Geometry check sheet. Reference: drawing and pictorial views, mm from the part's lowest x, y, z. A direction names the side the tool comes from. Give positions to 0.01 mm unless a question says otherwise; leave off trailing zeros. Write each loop counter-clockwise with the first axis right and the second up, starting at its lowest first coordinate (ties: lowest second). Pieces come first, ordered by that corner, then holes.
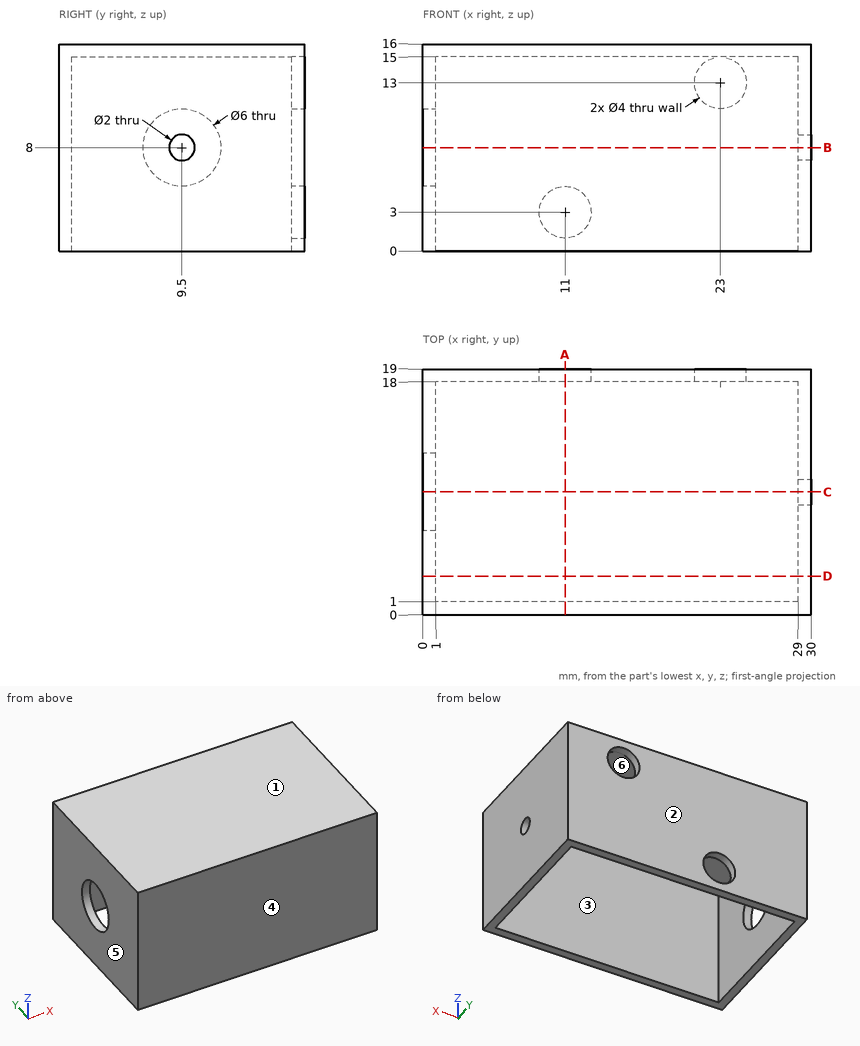
Item 1: Sectioned sample at C-C on y = 9.5. Record the cut outline in (x, z), then the cut area to 3 significant figures.
Answer key:
outline: (0, 0) - (1, 0) - (1, 5) - (0, 5) - close; (0, 11) - (1, 11) - (1, 15) - (29, 15) - (29, 9) - (30, 9) - (30, 16) - (0, 16) - close; (29, 0) - (30, 0) - (30, 7) - (29, 7) - close
area: 52.0 mm2
Item 2: Sectioned sample at D-D on y = 3. Record the cut outline in (x, z), then the cut area to 3 significant figures.
Answer key:
outline: (0, 0) - (1, 0) - (1, 15) - (29, 15) - (29, 0) - (30, 0) - (30, 16) - (0, 16) - close
area: 60.0 mm2
Item 3: Release check for a two-part mould opening along Y. For the marked faces 1, 2, 3 and 4 record: released by +Y, released by -Y, zero draft, split by the parting line, or undercut.
Answer key:
face 1: zero draft
face 2: released by +Y
face 3: undercut
face 4: released by -Y
Item 4: Scan lines: line 1 along X through (y, z) = (6.5, 13.5); line 2 along Y through (x, z) = (11.75, 14); line 3 along Y through (x, z) = (0.75, 8). Record each from-to range of solid material in increasing order.
Answer key:
line 1: x = 0 to 1, 29 to 30
line 2: y = 0 to 1, 18 to 19
line 3: y = 0 to 6.5, 12.5 to 19
Item 5: Sectioned sample at B-B on z = 8. Record the cut outline in (x, y).
Answer key:
outline: (0, 0) - (30, 0) - (30, 8.5) - (29, 8.5) - (29, 1) - (1, 1) - (1, 6.5) - (0, 6.5) - close; (0, 12.5) - (1, 12.5) - (1, 18) - (29, 18) - (29, 10.5) - (30, 10.5) - (30, 19) - (0, 19) - close
Item 6: Set-up check for the marked faces 5 and 6: record each of +Z, -Z, +X, -X, +Y, -Y from which the full face is reachable in a straight line by a thin tool's end or side.
Answer key:
face 5: +Z, -Z, -X, +Y, -Y
face 6: -Z
Item 7: Sectioned sample at A-A on x = 11. Record the cut outline in (y, z).
Answer key:
outline: (0, 0) - (1, 0) - (1, 15) - (18, 15) - (18, 5) - (19, 5) - (19, 16) - (0, 16) - close; (18, 0) - (19, 0) - (19, 1) - (18, 1) - close
